Read the model definition and answer for the solid it produces. Units are mm, in the model's axes. Coordinates: 2 decimals unless noted, no trailing zeros. Order: outer loops, then holes, each group sorted by start corner. A loop starts at its lowest first (then second) coordinate and runs counter-clockwise, first axis right, second up. Notation, with made-up numbers: (-21, 54) - (-5, 54) arc R8 cw to (-5, 67) - close; hole circle Ø8 at (58.25, 29.5). An arc over 180 degrees is marked (long way). Use one line per item in the form item = value.
```python
from build123d import *

# Parameters (mm, degrees)
SKETCH1_R           = 15
SKETCH1_R_2         = 13.5
BOSS_EXTRUDE1_DEPTH = 700
SKETCH2_W           = 30
SKETCH2_H           = 2.5
CUT_EXTRUDE1_DEPTH  = 2.5


with BuildPart() as part:
    # Sketch1 → Boss-Extrude1 (new body)
    with BuildSketch(Plane(origin=(0, 0, 0), x_dir=(1, 0, 0), z_dir=(0, 1, 0))):
        Circle(SKETCH1_R)
        Circle(SKETCH1_R_2, mode=Mode.SUBTRACT)
    extrude(amount=BOSS_EXTRUDE1_DEPTH)

    # Sketch2 → Cut-Extrude1 (cut)
    with BuildSketch(Plane(origin=(0, 700, 0), x_dir=(1, 0, 0), z_dir=(0, 1, 0))):
        Rectangle(SKETCH2_W, SKETCH2_H)
    extrude(amount=-CUT_EXTRUDE1_DEPTH, mode=Mode.SUBTRACT)


solid = part.part
```
(1) The mould has two halves that part along X. Classify faces 1 (the cylindrical face through (-14.985, 345.1, -0.66)), 2 (the cylindrical face through (-2.93, 345.1, 13.18)), 3 (the flat face through (0, 700, -14)): +X half, -X half, draft (parallel to the pull), parting line (faces both ways), or undercut.
Answer list:
face_1 = parting line
face_2 = undercut
face_3 = draft
(2) Straight lines are drawn through the part: L1, parallel to Z at x = 0, y = 460.5; L2, parallel to Z at x = 2, y = 104.5; L3, parallel to X at y = 586, z = 1. For each, find the intervals that lie inside material, in ascending order.
Answer list:
L1 = -15 to -13.5, 13.5 to 15
L2 = -14.87 to -13.35, 13.35 to 14.87
L3 = -14.97 to -13.46, 13.46 to 14.97
(3) Given pin 1 Ø3 at (x, y) = (7.5, 182) entering from -Z; pin 2 Ø1.2 at (x, y) = (-14, 699) entering from -Z; pin 3 Ø0.8 at (x, y) = (14, 698) entering from +Z, each flat-ended and moving along its own axis, determine where each tip first touches the part or whether it passes through.
Answer list:
pin_1 = -13.75
pin_2 = -6.74
pin_3 = 6.33
(4) Section B-B, the plane y = 91.5 is taken. Write down the section's boundary in (x, z), then the cut area to 3 significant figures.
Answer list:
outline = circle Ø30 at (0, 0); hole circle Ø27 at (0, 0)
area = 134 mm2
(5) Section A-A, the plane x = 0 is taken. Write down the section's boundary in (y, z).
Answer list:
outline = (0, -15) - (700, -15) - (700, -13.5) - (0, -13.5) - close; (0, 13.5) - (700, 13.5) - (700, 15) - (0, 15) - close
